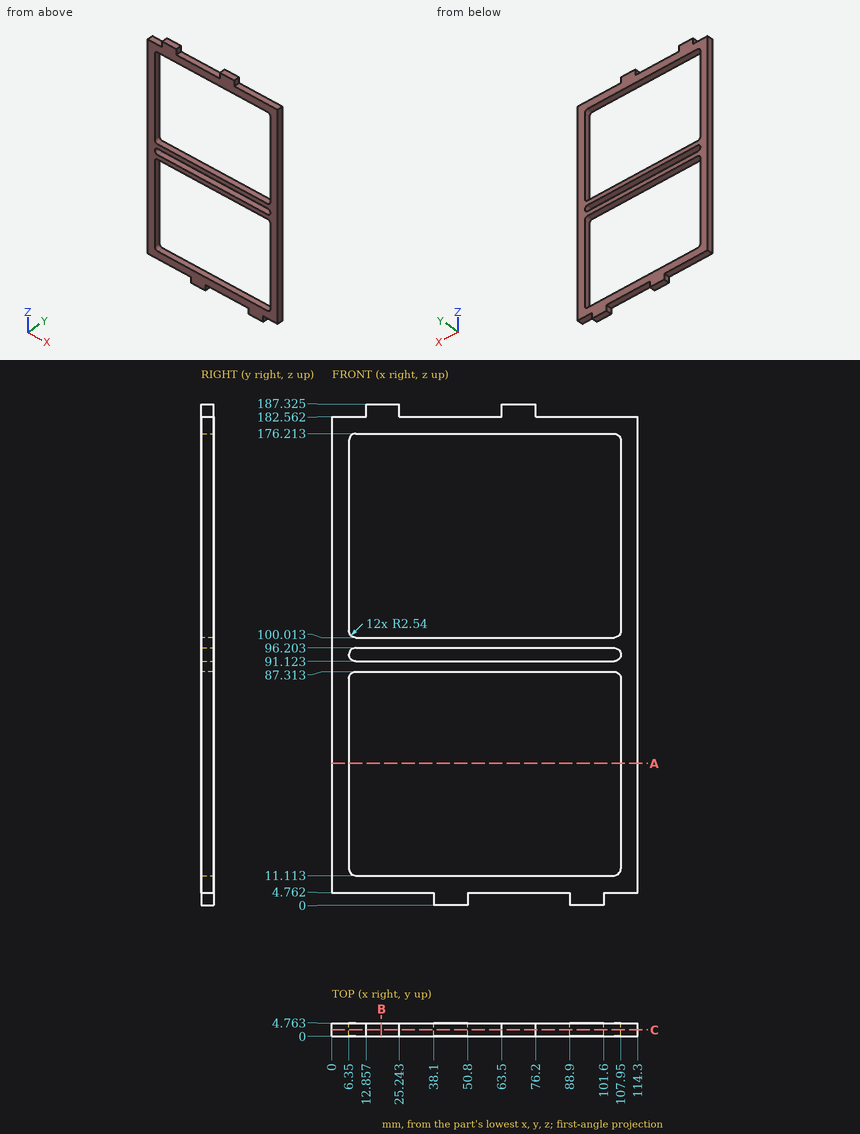
The figure shows three views and two pictorial views of one solid part (mm, origin at its lowest corner). Answer the questions. Round coordinates to 2 decimals unless told otherwise and drop trailing zeros. Order: outer loops, then holes, each group sorted by start corner. A loop starts at its lowest first (then second) coordinate and runs counter-clockwise, first axis right, second up. Notation, with made-up numbers: (26.5, 77.25) - (62.5, 77.25) arc R25 ccw to (62.5, 91.25) - close; hole circle Ø4 at (-14, -34.5). An arc over 180 degrees is marked (long way). Write item = value, one per line. Start each with the question number.
1) Section B-B, the plane x = 18.5 is taken. Write down the section's boundary in (y, z) (1 decimal).
2) Section A-A, the plane z = 53 is taken. Write down the section's boundary in (x, y).
3) Given pin 1 (2.5 mm diameter, centred on y = 1.5, z = 186, fed in from -X); pin 2 (1.4 mm diameter, centred on x = 45, y = 2, fed in from +Z); pin 3 (1.4 mm diameter, centred on x = 109, y = 3, fed in from -Z), each flat-ended and moving along its own axis, determine where each tip first touches the part or whether it passes through.
4) Straight lines are drawn through the part: L1, parallel to Z at x = 72.5, y = 0.7 (1 decimal); L2, parallel to Z at x = 30, y = 2.25; L3, parallel to X at y = 1.8, z = 62. For each, find the intervals that lie inside material, in ascending order.
5) Section C-C, the plane y = 2.25 is taken. Count the separate pieces of the cut face and the enclosed holes in it, plus the area to 3 significant figures.
Results list:
q1.outline = (0, 4.8) - (4.8, 4.8) - (4.8, 11.1) - (0, 11.1) - close; (0, 87.3) - (4.8, 87.3) - (4.8, 91.1) - (0, 91.1) - close; (0, 96.2) - (4.8, 96.2) - (4.8, 100) - (0, 100) - close; (0, 176.2) - (4.8, 176.2) - (4.8, 187.3) - (0, 187.3) - close
q2.outline = (0, 0) - (6.35, 0) - (6.35, 4.76) - (0, 4.76) - close; (107.95, 0) - (114.3, 0) - (114.3, 4.76) - (107.95, 4.76) - close
q3.pin_1 = 12.86
q3.pin_2 = 182.56
q3.pin_3 = 4.76
q4.L1 = 4.8 to 11.1, 87.3 to 91.1, 96.2 to 100, 176.2 to 187.3
q4.L2 = 4.76 to 11.11, 87.31 to 91.12, 96.2 to 100.01, 176.21 to 182.56
q4.L3 = 0 to 6.35, 107.95 to 114.3
q5.separate_pieces = 1
q5.enclosed_holes = 3
q5.area = 4,580 mm^2
